CAD build for the part. Positions are in the model's coordinates, mm. Face numbers are marked on the shaded views. A direction names the side the tool comes from. Give positions to 0.01 mm unless a question says otherwise; leave off trailing zeros. Loops run counter-clockwise (first coordinate to the right, second up) from the corner with the lowest first, then second, coordinate; pieces in that order, holes last. Notation, with made-up numbers: M 40.5,8 L 55.5,8 A26 ccw 55.5,42 Z; hole C 25,-32.5 d1. An arc over 180 degrees is marked long. Answer as CSV lines item,"result".
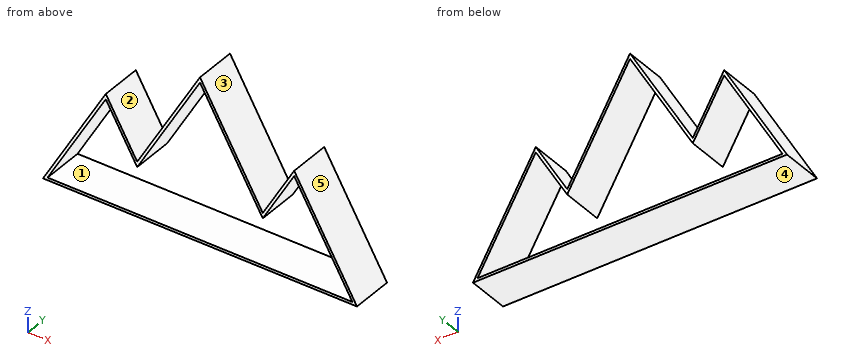
from build123d import *

# Parameters (mm, degrees)
F1_DEPTH = 101.6
F2_T     = -6.35
F4_DEPTH = 6.35


with BuildPart() as f1:
    # F0 (on Front) → F1 (new body)
    with BuildSketch(Plane.XZ):
        Polygon((152.4, 263.9645430735), (0, 0), (762, 0), (609.6, 263.9645430735), (533.4, 131.9822715367), (381, 395.9468146102), (228.6, 131.9822715367), align=None)
    extrude(amount=F1_DEPTH)

    # F2
    f2_openings = [f1.faces().sort_by_distance(p)[0] for p in [
        (381, -101.6, 120.250514),
    ]]
    offset(amount=F2_T, openings=f2_openings, kind=Kind.INTERSECTION)

    # F3 (on face) → F4 (cut)
    with BuildSketch(Plane.XZ.offset(6.35)):
        Polygon((152.4, 251.2645430735), (10.9985226281, 6.35), (751.0014773719, 6.35), (609.6, 251.2645430735), (533.4, 119.2822715367), (381, 383.2468146102), (228.6, 119.2822715367), align=None)
    extrude(amount=-F4_DEPTH, mode=Mode.SUBTRACT)


solid = f1.part
1) Band-saw the part on D-D on z = 102. Give the cut face in (x, y).
Answer below:
outline,"M 58.89,-101.6 L 66.22,-101.6 L 66.22,0 L 58.89,0 Z; M 695.78,-101.6 L 703.11,-101.6 L 703.11,0 L 695.78,0 Z"
2) Drill centre lines: line 1 (X direction, y = -67.5, z = 238.5); line 2 (X direction, y = -47, z = 211); line 3 (Z direction, x = 276, y = -9). Where is each one in solid material? Low to high. Write a range as from..to.
Answer below:
line 1,"x = 137.7..145.03, 159.77..167.1, 290.1..297.43, 464.57..471.9, 594.9..602.23, 616.97..624.3"
line 2,"x = 121.82..129.15, 175.65..182.98, 274.22..281.55, 480.45..487.78, 579.02..586.35, 632.85..640.18"
line 3,"z = 0..6.35, 201.38..214.08"
3) Band-saw the part on C-C on x = 358.5. Give the cut face in (y, z).
Answer below:
outline,"M -101.6,0 L 0,0 L 0,6.35 L -101.6,6.35 Z; M -101.6,344.28 L 0,344.28 L 0,356.98 L -101.6,356.98 Z"
4) Which spindle directions (+Z, -Z, +X, -X, +Y, -Y) get a long thin tool onto all of the face, cutting with end or side? Do the marked faces 1 and 2. Say none if no direction does.
Answer below:
face 1,"+Y, -Y"
face 2,"+Z, +Y, -Y"
5) Flat gauge pins, fed straight in: pin 1 (10 mm diameter, centred on y = -17, z = 40, fed in from -X); pin 2 (10 mm diameter, centred on x = 587.5, y = -45.5, fed in from +Z); pin 3 (1.5 mm diameter, centred on x = 327, y = -66.5, fed in from +Z). Where does each tip first touch, or does it go through?
Answer below:
pin 1,"stops at x = 20.21"
pin 2,"stops at z = 234.35"
pin 3,"stops at z = 303.72"
6) Mould opens along X. For the marked faces 3, 4 and 5 say: +X half, -X half, draft (parallel to the pull), parting line (faces both ways), or undercut.
Answer below:
face 3,"undercut"
face 4,"draft"
face 5,"+X half"
7) Band-saw the part on A-A on y = -27. Give the cut face in (x, z), and give its area (3 significant figures).
Answer below:
outline,"M 0,0 L 762,0 L 609.6,263.96 L 533.4,131.98 L 381,395.95 L 228.6,131.98 L 152.4,263.96 Z; hole M 11,6.35 L 751,6.35 L 609.6,251.26 L 533.4,119.28 L 381,383.25 L 228.6,119.28 L 152.4,251.26 Z"
area,"14,300 mm^2"
8) Band-saw the part on B-B on z = 163. Give the cut face in (x, y), and give its area (3 significant figures).
Answer below:
outline,"M 94.11,-101.6 L 101.44,-101.6 L 101.44,0 L 94.11,0 Z; M 203.36,-101.6 L 210.69,-101.6 L 210.69,0 L 203.36,0 Z; M 246.51,-101.6 L 253.84,-101.6 L 253.84,0 L 246.51,0 Z; M 508.16,-101.6 L 515.49,-101.6 L 515.49,0 L 508.16,0 Z; M 551.31,-101.6 L 558.64,-101.6 L 558.64,0 L 551.31,0 Z; M 660.56,-101.6 L 667.89,-101.6 L 667.89,0 L 660.56,0 Z"
area,"4,470 mm^2"
